Verification items for this drawing (mm, ordinates from the low corner). A direction names the side the tool comes from. Coordinates: 2 decimals unless noted, no trailing zeros. Write each loop counter-clockwise with the first axis right and the second up, starting at its lowest first coordinate (ties: lowest second). Pieces come first, ordered by that corner, then holes. Notation, with made-up numbers: (89, 1.25) -> (98, 1.25) arc R37 cw to (98, 39.25) -> close; hole circle Ø1 at (-1.5, 69). An arc over 180 degrees is marked (long way). Put each result on its own line as item: value. Start each with the question number.
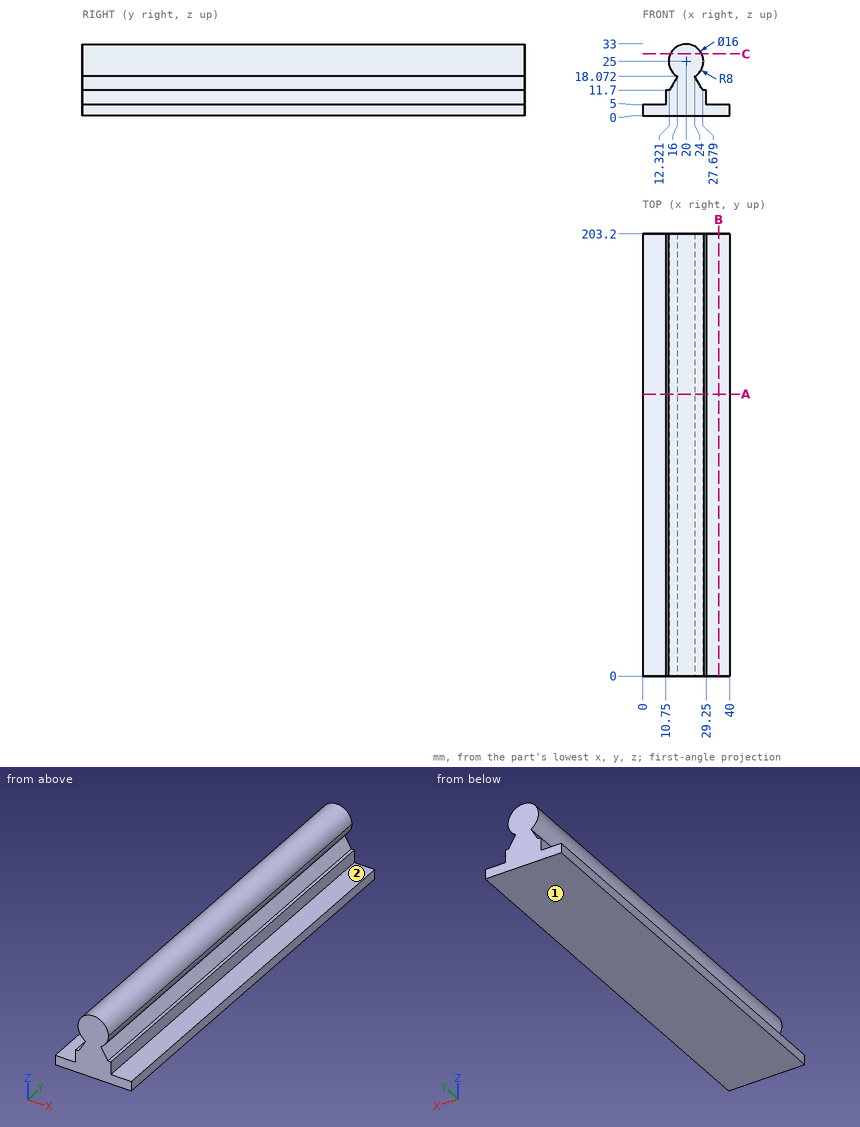
Item 1: Section check A-A, the plane y = 129.5. Enter the section's corners in (x, z), and give its area (3 significant figures).
Item 2: Scan lines: line 1 along Z through (x, y) = (8, 57); line 2 along X through (y, z) = (133, 7); line 3 along X through (y, z) = (188.5, 18). Record each from-to range of solid material in increasing order. Write a range as [from, to].
Item 3: Go/stop test with flat-tipped pins: P1, Ø3.5, axis at y = 108.5, z = 8, coming from the +X side; P2, Ø10, axis at y = 129, z = 17, coming from the -X side (1 decimal); P3, Ø1.7, axis at x = 28, y = 107, coming from the +Z side. Record where each tip stops, or that it passes through.
Item 4: Section check C-C, the plane z = 28.5. Enter the section's corners in (x, y), and give its area (3 significant figures).
Item 5: Access from +Z, -Z, +X, -X, +Y, -Y to the whole of each face (thin tool, end or side, straight path). Record for the marked faces 1 and 2.
Item 6: Section check B-B, the plane x = 35. Enter the section's corners in (y, z).
From the geometry:
1. outline: (0, 0) -> (40, 0) -> (40, 5) -> (29.25, 5) -> (29.25, 11.7) -> (27.68, 11.7) -> (24, 18.07) arc R8 ccw (long way) to (16, 18.07) -> (12.32, 11.7) -> (10.75, 11.7) -> (10.75, 5) -> (0, 5) -> close
1. area: 594 mm²
2. line 1: [0, 5]
2. line 2: [10.75, 29.25]
2. line 3: [15.96, 24.04]
3. P1: x = 29.25
3. P2: x = 12.5
3. P3: z = 28.59
4. outline: (12.81, 0) -> (27.19, 0) -> (27.19, 203.2) -> (12.81, 203.2) -> close
4. area: 2,920 mm²
5. face 1: -Z, +X, -X, +Y, -Y
5. face 2: +Z, +X, +Y, -Y
6. outline: (0, 0) -> (203.2, 0) -> (203.2, 5) -> (0, 5) -> close
